Design review of the part built by this model. Coordinates are the model's own, in mm. Round coordinates to 2 decimals unless told otherwise and drop trailing zeros. Loops run counter-clockwise (first coordinate to the right, second up) from the corner with the lowest first, then second, coordinate; pieces in that order, holes last. Notation, with made-up numbers: (9, 29.5) - (63, 29.5) arc R27 cw to (63, 67.5) - close; hole circle Ø8 at (17, -33). An arc over 180 degrees is marked (long way). Return JSON: item names as keys, results as strings. Group by question number.
from build123d import *

# Parameters (mm, degrees)
F0_R     = 44.45
F0_W     = 3.3813905481
F0_H     = 17.2546718104
F1_DEPTH = 6.35


with BuildPart() as f1:
    # F0 (on Front) → F1 (new body)
    with BuildSketch(Plane.XZ):
        Circle(F0_R)
        with BuildLine():
            Line((-27.5039295863, -2.7326104788), (-29.3312287807, -2.7326104788))
            Line((-29.3312287807, -2.7326104788), (-29.3312287807, -8.9525240473))
            Line((-29.3312287807, -8.9525240473), (-32.7693897892, -8.9525240473))
            Line((-32.7693897892, -8.9525240473), (-32.7693897892, 7.2589905531))
            Line((-32.7693897892, 7.2589905531), (-28.046797114, 7.2589905531))
            add(Edge.make_bspline(
                [(-28.046797114, 7.2589905531), (-24.7399177952, 7.2589905531), (-23.1556671344, 6.0561664231)],
                knots=[0, 0, 0, 1, 1, 1], degree=2))
            add(Edge.make_bspline(
                [(-23.1556671344, 6.0561664231), (-21.5714164736, 4.8533422932), (-21.5714164736, 2.4015680344)],
                knots=[0, 0, 0, 1, 1, 1], degree=2))
            add(Edge.make_bspline(
                [(-21.5714164736, 2.4015680344), (-21.5714164736, 0.9716620628), (-22.3573325349, -0.1424582227)],
                knots=[0, 0, 0, 1, 1, 1], degree=2))
            add(Edge.make_bspline(
                [(-22.3573325349, -0.1424582227), (-23.1432485962, -1.2565785082), (-24.5873471828, -1.8881498803)],
                knots=[0, 0, 0, 1, 1, 1], degree=2))
            add(Edge.make_bspline(
                [(-24.5873471828, -1.8881498803), (-20.9256524865, -7.3558548484), (-19.8186285085, -8.9525240473)],
                knots=[0, 0, 0, 1, 1, 1], degree=2))
            Line((-19.8186285085, -8.9525240473), (-23.6328938172, -8.9525240473))
            Line((-23.6328938172, -8.9525240473), (-27.5039295863, -2.7326104788))
        make_face(mode=Mode.SUBTRACT)
        with BuildLine():
            add(Edge.make_bspline(
                [(-7.5100830612, 0.6718430688), (-6.7791633834, -0.7811259023), (-6.7791633834, -2.7326104788)],
                knots=[0, 0, 0, 1, 1, 1], degree=2))
            add(Edge.make_bspline(
                [(-6.7791633834, -2.7326104788), (-6.7791633834, -5.7591856494), (-8.3758325824, -7.4676216923)],
                knots=[0, 0, 0, 1, 1, 1], degree=2))
            add(Edge.make_bspline(
                [(-8.3758325824, -7.4676216923), (-9.9725017814, -9.1760577352), (-12.8216692632, -9.1760577352)],
                knots=[0, 0, 0, 1, 1, 1], degree=2))
            add(Edge.make_bspline(
                [(-12.8216692632, -9.1760577352), (-14.6063906122, -9.1760577352), (-15.9706557389, -8.3936898277)],
                knots=[0, 0, 0, 1, 1, 1], degree=2))
            add(Edge.make_bspline(
                [(-15.9706557389, -8.3936898277), (-17.3349208656, -7.6113219202), (-18.0658405434, -6.1477084878)],
                knots=[0, 0, 0, 1, 1, 1], degree=2))
            add(Edge.make_bspline(
                [(-18.0658405434, -6.1477084878), (-18.7967602211, -4.6840950554), (-18.7967602211, -2.7326104788)],
                knots=[0, 0, 0, 1, 1, 1], degree=2))
            add(Edge.make_bspline(
                [(-18.7967602211, -2.7326104788), (-18.7967602211, 0.304609153), (-17.2125095604, 1.9899821964)],
                knots=[0, 0, 0, 1, 1, 1], degree=2))
            add(Edge.make_bspline(
                [(-17.2125095604, 1.9899821964), (-15.6282588996, 3.6753552398), (-12.7542543414, 3.6753552398)],
                knots=[0, 0, 0, 1, 1, 1], degree=2))
            add(Edge.make_bspline(
                [(-12.7542543414, 3.6753552398), (-10.9695329923, 3.6753552398), (-9.6052678656, 2.9000836398)],
                knots=[0, 0, 0, 1, 1, 1], degree=2))
            add(Edge.make_bspline(
                [(-9.6052678656, 2.9000836398), (-8.2410027389, 2.1248120399), (-7.5100830612, 0.6718430688)],
                knots=[0, 0, 0, 1, 1, 1], degree=2))
        make_face(mode=Mode.SUBTRACT)
        with Locations((-2.2925229343, -0.3251881421)):
            Rectangle(F0_W, F0_H, mode=Mode.SUBTRACT)
        with Locations((4.6370213893, -0.3251881421)):
            Rectangle(F0_W, F0_H, mode=Mode.SUBTRACT)
        with BuildLine():
            add(Edge.make_bspline(
                [(17.9479202783, -8.9596203549), (16.940244606, -9.1760577352), (15.485501558, -9.1760577352)],
                knots=[0, 0, 0, 1, 1, 1], degree=2))
            add(Edge.make_bspline(
                [(15.485501558, -9.1760577352), (12.4944079253, -9.1760577352), (10.8090348819, -7.5226180758)],
                knots=[0, 0, 0, 1, 1, 1], degree=2))
            add(Edge.make_bspline(
                [(10.8090348819, -7.5226180758), (9.1236618385, -5.8691784164), (9.1236618385, -2.8426032459)],
                knots=[0, 0, 0, 1, 1, 1], degree=2))
            add(Edge.make_bspline(
                [(9.1236618385, -2.8426032459), (9.1236618385, 0.272675769), (10.681301346, 1.9740155044)],
                knots=[0, 0, 0, 1, 1, 1], degree=2))
            add(Edge.make_bspline(
                [(10.681301346, 1.9740155044), (12.2389408534, 3.6753552398), (14.9887600295, 3.6753552398)],
                knots=[0, 0, 0, 1, 1, 1], degree=2))
            add(Edge.make_bspline(
                [(14.9887600295, 3.6753552398), (17.6143938234, 3.6753552398), (19.0780072558, 2.1798084234)],
                knots=[0, 0, 0, 1, 1, 1], degree=2))
            add(Edge.make_bspline(
                [(19.0780072558, 2.1798084234), (20.5416206882, 0.684261607), (20.5416206882, -1.955564802)],
                knots=[0, 0, 0, 1, 1, 1], degree=2))
            Line((20.5416206882, -1.955564802), (20.5416206882, -3.5983600001))
            Line((20.5416206882, -3.5983600001), (12.5476302319, -3.5983600001))
            add(Edge.make_bspline(
                [(12.5476302319, -3.5983600001), (12.6044006923, -5.0389104329), (13.4027352918, -5.8478894938)],
                knots=[0, 0, 0, 1, 1, 1], degree=2))
            add(Edge.make_bspline(
                [(13.4027352918, -5.8478894938), (14.2010698913, -6.6568685546), (15.6416203242, -6.6568685546)],
                knots=[0, 0, 0, 1, 1, 1], degree=2))
            add(Edge.make_bspline(
                [(15.6416203242, -6.6568685546), (16.7628369172, -6.6568685546), (17.7598681281, -6.4244644823)],
                knots=[0, 0, 0, 1, 1, 1], degree=2))
            add(Edge.make_bspline(
                [(17.7598681281, -6.4244644823), (18.7568993391, -6.19206041), (19.8426343944, -5.6811262663)],
                knots=[0, 0, 0, 1, 1, 1], degree=2))
            Line((19.8426343944, -5.6811262663), (19.8426343944, -8.2996637526))
            add(Edge.make_bspline(
                [(19.8426343944, -8.2996637526), (18.9555959505, -8.7431829746), (17.9479202783, -8.9596203549)],
                knots=[0, 0, 0, 1, 1, 1], degree=2))
        make_face(mode=Mode.SUBTRACT)
        with BuildLine():
            add(Edge.make_bspline(
                [(28.0761252305, 3.0384616371), (29.0571897494, 3.6753552398), (30.2103397265, 3.6753552398)],
                knots=[0, 0, 0, 1, 1, 1], degree=2))
            add(Edge.make_bspline(
                [(30.2103397265, 3.6753552398), (30.8986815589, 3.6753552398), (31.3528452422, 3.5760069341)],
                knots=[0, 0, 0, 1, 1, 1], degree=2))
            Line((31.3528452422, 3.5760069341), (31.0973781704, 0.4075056125))
            add(Edge.make_bspline(
                [(31.0973781704, 0.4075056125), (30.6857923324, 0.5174983795), (30.1003469594, 0.5174983795)],
                knots=[0, 0, 0, 1, 1, 1], degree=2))
            add(Edge.make_bspline(
                [(30.1003469594, 0.5174983795), (28.4823888378, 0.5174983795), (27.577609625, -0.3145436808)],
                knots=[0, 0, 0, 1, 1, 1], degree=2))
            add(Edge.make_bspline(
                [(27.577609625, -0.3145436808), (26.6728304123, -1.1465857412), (26.6728304123, -2.6439066345)],
                knots=[0, 0, 0, 1, 1, 1], degree=2))
            Line((26.6728304123, -2.6439066345), (26.6728304123, -8.9525240473))
            Line((26.6728304123, -8.9525240473), (23.2914398642, -8.9525240473))
            Line((23.2914398642, -8.9525240473), (23.2914398642, 3.4447252444))
            Line((23.2914398642, 3.4447252444), (25.8532068901, 3.4447252444))
            Line((25.8532068901, 3.4447252444), (26.3534965725, 1.3584108243))
            Line((26.3534965725, 1.3584108243), (26.5167116462, 1.3584108243))
            add(Edge.make_bspline(
                [(26.5167116462, 1.3584108243), (27.0950607116, 2.4015680344), (28.0761252305, 3.0384616371)],
                knots=[0, 0, 0, 1, 1, 1], degree=2))
        make_face(mode=Mode.SUBTRACT)
    extrude(amount=F1_DEPTH)


solid = f1.part
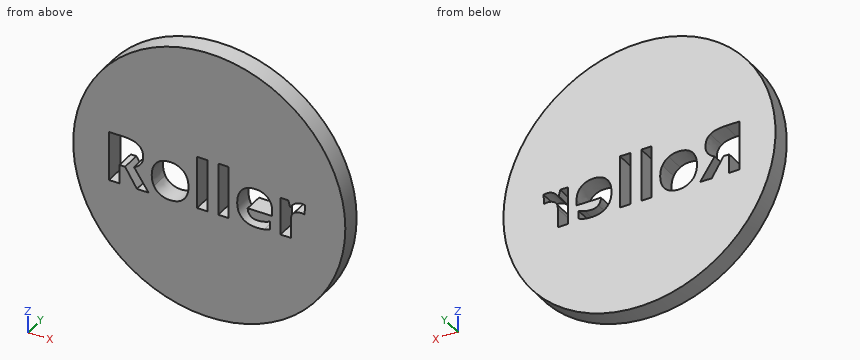
Q1. Add section B-B, the plane y = -4.25. Give the number of separate pieces and of enclosed holes in the cut face, plus the area to 3 significant figures.
Q2. Add section C-C, the plane z = -19.5. State the section outline as (x, y) points, plus the area to 3 significant figures.
Q3. Add section D-D, the plane z = -36. State the section outline as (x, y) points, plus the area to 3 significant figures.
Q4. Add section A-A, the plane x = -30.5. State the section outline as (y, z) points (3 decimals), plus the area to 3 significant figures.
Q5. Insertion check: pin 1 Ø1.5 at (x, y) = (3.5, -5.5) entering from +Z; pin 2 Ø1.7 at (x, y) = (-2, -2.5) entering from -Z; pin 3 Ø1.8 at (y, z) = (-3, -3) entering from -X. Each pin has a flat end and moves straight along its axis. Give the tip position at first contact, or say it passes through.
Q6. For line 1 (Z direction, x = 4.5, y = -2); line 2 (Z direction, x = -28, y = -3.5); line 3 (Z direction, x = -19.5, y = -4.5), list the stretches that pass through material, from the lowest coordinate up.
Evaluation:
{
 "1": {"separate pieces": "1", "enclosed holes": "6", "area": "5,660 mm²"},
 "2": {"outline": "(-39.94, -6.35) - (39.94, -6.35) - (39.94, 0) - (-39.94, 0) - close", "area": "507 mm²"},
 "3": {"outline": "(-26.07, -6.35) - (26.07, -6.35) - (26.07, 0) - (-26.07, 0) - close", "area": "331 mm²"},
 "4": {"outline": "(-6.35, -32.335) - (0, -32.335) - (0, -8.953) - (-6.35, -8.953) - close; (-6.35, 7.259) - (0, 7.259) - (0, 32.335) - (-6.35, 32.335) - close", "area": "308 mm²"},
 "5": {"pin 1": "z = 44.36", "pin 2": "z = -44.44", "pin 3": "x = -44.4"},
 "6": {"line 1": "-44.22 to -8.95, 8.3 to 44.22", "line 2": "-34.52 to -2.73, 7.26 to 34.52", "line 3": "-39.94 to 39.94"}
}
